Check sheet for the modelled part. Datum: model origin and axes. Units: mm. A direction names the side the tool comes from. Round coordinates to 2 decimals unless told otherwise and drop trailing zeros. Order: outer loops, then holes, each group sorted by start corner. A loop starts at its lowest first (then second) coordinate and runs counter-clockwise, first axis right, second up.
Q1. Cross-section at C-C on z = 166.5. Record the cut outline in (x, y).
Q2. Set-up check for faces 4 (the flat face through (-30.5, 30, 154)), 5 (the cylindrical face through (5.77, -11.09, 226.47)), 6 (the cylindrical face through (5.77, -11.09, 24.65)), 7 (the flat face through (0, 17, 142.56)): record each of +Z, -Z, +X, -X, +Y, -Y from which the full face is reachable in a straight line by a thin tool's end or side.
Q3. Cross-section at B-B on y = -35.5. Record the cut outline in (x, z), then the cut area to 3 significant figures.
Q4. Depth check by flat-ended pin: P1, Ø2.5, axis at x = 0, z = 19, coming from the +Y side; P2, Ø6, axis at x = -37.5, z = 91, coming from the -Y side; P3, Ø5.5, axis at y = 27, z = 96.5, coming from the +X side. Enter the tip coordinate at first touch or a pass-through.
Q5. Scan lines: probe 1 along Z at (x, y) = (4.5, 9); probe 2 along Z at (x, y) = (5.5, -51); probe 3 along X at (y, z) = (22, 159.5). Record each from-to range of solid material in increasing order.
Q6. Mould release check, pull along Z, two halves, no side actions. Record for faces 1 (the flat face through (-3.4, 12.3, 201.12)), 2 (the flat face through (4, 6, 22)), 3 (the cylindrical face through (-14.985, 0.66, 57.395)): +Z half, -Z half, draft (parallel to the pull), parting line (faces both ways), or undercut.
Q7. Cross-section at A-A on x = -37. Record the cut outline in (y, z).
from build123d import *
from build123d.topology import SkipClean

# Parameters (mm, degrees)
SKETCH1_R                = 12.5
BOSS_EXTRUDE1_DEPTH      = 50
SKETCH2_R                = 15
BOSS_EXTRUDE2_DEPTH      = 15
SKETCH3_R                = 22.5
BOSS_EXTRUDE3_DEPTH      = 23
BOSS_EXTRUDE4_DEPTH      = 18.56
BOSS_EXTRUDE5_DEPTH      = 60
BOSS_EXTRUDE5_DEPTH_BACK = 60
CUT_EXTRUDE1_DEPTH       = 29.78
CUT_EXTRUDE2_DEPTH       = 59.56
SKETCH9_R                = 25.5
BOSS_EXTRUDE7_DEPTH      = 2
SKETCH10_R               = 22.5
BOSS_EXTRUDE8_DEPTH      = 17
CUT_EXTRUDE3_DEPTH       = 17


with BuildPart() as part:
    # Sketch1 → Boss-Extrude1 (new body)
    with BuildSketch(Plane.XY):
        Circle(SKETCH1_R)
    extrude(amount=BOSS_EXTRUDE1_DEPTH)

    # Sketch2 → Boss-Extrude2 (add)
    with BuildSketch(Plane.XY.offset(50)):
        Circle(SKETCH2_R)
    extrude(amount=BOSS_EXTRUDE2_DEPTH)

    # Sketch3 → Boss-Extrude3 (add)
    with BuildSketch(Plane.XY.offset(65)):
        Circle(SKETCH3_R)
    extrude(amount=BOSS_EXTRUDE3_DEPTH)

    # Sketch4 → Boss-Extrude4 (add)
    with BuildSketch(Plane.XY.offset(88)):
        with BuildLine():
            Line((-57.076702778, -18.5), (57.076702778, -18.5))
            ThreePointArc((57.076702778, -18.5), (0, -60), (-57.076702778, -18.5))
        make_face()
    extrude(amount=BOSS_EXTRUDE4_DEPTH)

    # Sketch5 → Boss-Extrude5 (add, two sides: drawn at the far end of the back side and taken through both)
    with BuildSketch(Plane(origin=(0, 0, 0), x_dir=(0, 0, -1), z_dir=(1, 0, 0)).offset(-BOSS_EXTRUDE5_DEPTH_BACK)):
        with BuildLine():
            Line((-106.56, -18.5), (-106.56, 70.5))
            Line((-106.56, 70.5), (-90.067236991, 70.5))
            ThreePointArc((-90.067236991, 70.5), (-88.075811945, 26.022247339), (-88, -18.5))
            Line((-88, -18.5), (-106.56, -18.5))
        make_face()
    extrude(amount=BOSS_EXTRUDE5_DEPTH + BOSS_EXTRUDE5_DEPTH_BACK)

    # Sketch7 → Cut-Extrude1 (cut, symmetric)
    with SkipClean():  # the faces are left unmerged after this step: merging them gives an invalid solid
        with BuildSketch(Plane(origin=(0, 0, 88), x_dir=(-1, 0, 0), z_dir=(0, 0, -1))):
            with BuildLine():
                Line((-60, 0), (-60, -18.5))
                Line((-60, -18.5), (-57.076702778, -18.5))
                ThreePointArc((-57.076702778, -18.5), (-59.264669773, -9.364769974), (-60, 0))
            make_face()
            with BuildLine():
                Line((60, 0), (60, -18.5))
                Line((60, -18.5), (57.076702778, -18.5))
                ThreePointArc((57.076702778, -18.5), (59.264669773, -9.364769974), (60, 0))
            make_face()
        extrude(amount=CUT_EXTRUDE1_DEPTH, both=True, mode=Mode.SUBTRACT)

    # Sketch8 → Cut-Extrude2 (cut)
    with SkipClean():  # the faces are left unmerged after this step: merging them gives an invalid solid
        with BuildSketch(Plane.XY.offset(106.56)):
            with BuildLine():
                Line((60, 70.5), (2.15e-07, 70.5))
                ThreePointArc((2.15e-07, 70.5), (21.565678046, 61.567835553), (30.499999847, 40.003051391))
                Line((30.499999847, 40.003051391), (30.499999847, 20.003051391))
                Line((30.499999847, 20.003051391), (60, 0))
                Line((60, 0), (60, 70.5))
            make_face()
            with BuildLine():
                Line((-60, 70.5), (-60, 0))
                Line((-60, 0), (-30.499999847, 20.003051391))
                Line((-30.499999847, 20.003051391), (-30.499999847, 40.003051391))
                ThreePointArc((-30.499999847, 40.003051391), (-21.565677894, 61.567835705), (2.15e-07, 70.5))
                Line((2.15e-07, 70.5), (-60, 70.5))
            make_face()
        extrude(amount=-CUT_EXTRUDE2_DEPTH, mode=Mode.SUBTRACT)

    # Sketch9 → Boss-Extrude7 (add)
    with SkipClean():  # the faces are left unmerged after this step: merging them gives an invalid solid
        with BuildSketch(Plane.XY.offset(106.56)):
            with Locations((0, 40)):
                Circle(SKETCH9_R)
        extrude(amount=BOSS_EXTRUDE7_DEPTH)

    # Sketch10 → Boss-Extrude8 (add)
    with SkipClean():  # the faces are left unmerged after this step: merging them gives an invalid solid
        with BuildSketch(Plane.XY.offset(108.56)):
            with Locations((0, 40)):
                Circle(SKETCH10_R)
        extrude(amount=BOSS_EXTRUDE8_DEPTH)

    # Sketch11 → Cut-Extrude3 (cut)
    with SkipClean():  # the faces are left unmerged after this step: merging them gives an invalid solid
        with BuildSketch(Plane(origin=(0, 0, 0), x_dir=(1, 0, 0), z_dir=(0, 1, 0))):
            with BuildLine():
                Line((4, -15), (4, -30))
                ThreePointArc((4, -30), (0, -34), (-4, -30))
                Line((-4, -30), (-4, -15))
                ThreePointArc((-4, -15), (0, -11), (4, -15))
            make_face()
        extrude(amount=CUT_EXTRUDE3_DEPTH, mode=Mode.SUBTRACT)

    # Mirror1: part across plane


with BuildPart() as part_1:
    with SkipClean():  # the faces are left unmerged after this step: merging them gives an invalid solid
        add(part.part)
        add(part.part.mirror(Plane(origin=(0, 40, 125.56), x_dir=(1, 0, 0), z_dir=(0, 0, 1))))


solid = part_1.part
Results found:
1. outline: circle Ø45 at (0, 0)
2. face 4: +Z, -Z, -X, +Y
2. face 5: +Z
2. face 6: -Z
2. face 7: none
3. outline: (-48.37, 88) - (48.37, 88) - (48.37, 106.56) - (-48.37, 106.56) - close; (-48.37, 144.56) - (48.37, 144.56) - (48.37, 163.12) - (-48.37, 163.12) - close
3. area: 3,590 mm2
4. P1: stops at y = 0
4. P2: stops at y = -49.09
4. P3: stops at x = 30.5
5. probe 1: z = 0 to 106.56, 144.56 to 251.12
5. probe 2: z = 88 to 106.56, 144.56 to 163.12
5. probe 3: x = -30.5 to 30.5
6. face 1: +Z half
6. face 2: undercut
6. face 3: draft
7. outline: (-47.23, 88) - (-18.5, 88) arc R1034.5 ccw to (15.6, 87.89) - (15.6, 106.56) - (-47.23, 106.56) - close; (-47.23, 144.56) - (15.6, 144.56) - (15.6, 163.23) arc R1034.5 ccw to (-18.5, 163.12) - (-47.23, 163.12) - close
